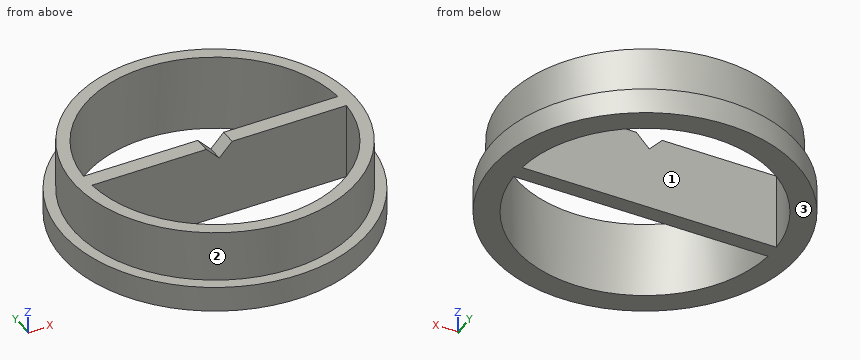
```python
from build123d import *

# Parameters (mm, degrees)
F0_R     = 7.531741
F0_R_2   = 6.35
F1_DEPTH = 1.27
F2_R     = 6.97558
F2_R_2   = 6.35
F3_DEPTH = 2.54
F5_W     = 13.57171
F5_H     = 0.779712
F6_DEPTH = 3.81
F8_DEPTH = 2.54


with BuildPart() as f1:
    # F0 (on Top) → F1 (new body)
    with BuildSketch(Plane.XY):
        Circle(F0_R)
        Circle(F0_R_2, mode=Mode.SUBTRACT)
    extrude(amount=F1_DEPTH)

    # F2 (on face) → F3 (join)
    with BuildSketch(Plane.XY.offset(1.27)):
        Circle(F2_R)
        Circle(F2_R_2, mode=Mode.SUBTRACT)
    extrude(amount=F3_DEPTH)

    # F5 (on face) → F6 (join)
    with BuildSketch(Plane.XY.offset(3.81)):
        Rectangle(F5_W, F5_H)
    extrude(amount=-F6_DEPTH)

    # F7 (on face) → F8 (cut)
    with BuildSketch(Plane.XZ.offset(0.389856)):
        Polygon((0.642504, 3.81), (0, 3.81), (0, 3.132625), align=None)
        Polygon((0, 3.132625), (0, 3.81), (-0.644351, 3.81), align=None)
    extrude(amount=-F8_DEPTH, mode=Mode.SUBTRACT)


solid = f1.part
```
Source: CAD feature listing. Evaluate the final solid. Frame: model axes, mm. Face numbers are marked on the shaded views. Give positions to 0.01 mm unless a question says otherwise; leave off trailing zeros. Order: outer loops, then holes, each group sorted by start corner. A loop starts at its lowest first (then second) coordinate and runs counter-clockwise, first axis right, second up.
(1) Section query D-D (y = 3.75). Return the cut outline in (x, z).
(2) Contact query for flat-ended pins moving along their axis: P1, Ø2, axis at x = -6, y = -1, coming from the +Z side; P2, Ø1, axis at x = 6, z = 2.5, coming from the -Y side. Output: stop coordinate, or through.
(3) Section query B-B (x = 2.5). Return the cut outline in (y, z).
(4) Section query C-C (y = 0). Return the cut outline in (x, z), plus the area to 3 significant figures.
(5) Section query A-A (z = 2.8). Return the cut outline in (x, y).
(6) Material intervals for line 1 along Y through (x, z) = (0, 0.55); line 2 along Y through (x, z) = (-2, 3.6); line 3 along X through (y, z) = (5.5, 2.55), sorted ascending.
(7) Pull-direction query (Y, two-part tool) for the marked faces 1, 2 and 3; classes: +Y half, -Y half, draft (parallel to the pull), parting line (faces both ways), or undercut.
Outcome:
1. outline: (-6.53, 0) - (-5.12, 0) - (-5.12, 3.81) - (-5.88, 3.81) - (-5.88, 1.27) - (-6.53, 1.27) - close; (5.12, 0) - (6.53, 0) - (6.53, 1.27) - (5.88, 1.27) - (5.88, 3.81) - (5.12, 3.81) - close
2. P1: stops at z = 3.81
2. P2: stops at y = -4.29
3. outline: (-7.1, 0) - (-5.84, 0) - (-5.84, 3.81) - (-6.51, 3.81) - (-6.51, 1.27) - (-7.1, 1.27) - close; (-0.39, 0) - (0.39, 0) - (0.39, 3.81) - (-0.39, 3.81) - close; (5.84, 0) - (7.1, 0) - (7.1, 1.27) - (6.51, 1.27) - (6.51, 3.81) - (5.84, 3.81) - close
4. outline: (-7.53, 0) - (7.53, 0) - (7.53, 1.27) - (6.98, 1.27) - (6.98, 3.81) - (0.64, 3.81) - (0, 3.13) - (-0.64, 3.81) - (-6.98, 3.81) - (-6.98, 1.27) - (-7.53, 1.27) - close
4. area: 54.1 mm2
5. outline: circle Ø13.95 at (0, 0); hole (-6.34, -0.39) arc R6.35 ccw to (6.34, -0.39) - close; hole (-6.34, 0.39) - (6.34, 0.39) arc R6.35 ccw to start
6. line 1: y = -7.53 to -6.35, -0.39 to 0.39, 6.35 to 7.53
6. line 2: y = -6.68 to -6.03, -0.39 to 0.39, 6.03 to 6.68
6. line 3: x = -4.29 to -3.17, 3.17 to 4.29
7. face 1: undercut
7. face 2: parting line
7. face 3: draft
